Model file for the job. Use its own axes, mm. A direction names the side the tool comes from. Give positions to 0.01 mm unless a question says otherwise; leave off trailing zeros. Write each loop counter-clockwise with the first axis right and the second up, starting at its lowest first coordinate (ties: lowest second). Pieces come first, ordered by that corner, then holes. Notation, with made-up numbers: (27.25, -38.5) - (45.25, -38.5) arc R14 cw to (45.25, -30.5) - close; hole circle Ø11 at (-39.5, -27.5). An arc over 180 degrees is marked (long way). Use a Markdown table: item, result. Add a question column.
```python
from build123d import *

# Parameters (mm, degrees)
F1_DEPTH = 63.5
F0_W     = 25.4
F0_H     = 19.05
F2_DEPTH = 25.4
F3_DEPTH = 7.9375
F5_R     = 15.875


with BuildPart() as f1:
    # F0 (on Front) → F1 (new body, symmetric)
    with BuildSketch(Plane.XZ):
        Polygon((41.275, -9.525), (41.275, 9.525), (22.225, 9.525), (-41.275, 9.525), (-41.275, -9.525), align=None)
    extrude(amount=F1_DEPTH, both=True)

    # F0 (on Front) → F2 (join, symmetric)
    with BuildSketch(Plane.XZ):
        Polygon((41.275, -9.525), (41.275, 9.525), (22.225, 9.525), (-41.275, 9.525), (-41.275, -9.525), align=None)
        with BuildLine():
            Line((22.225, 9.525), (41.275, 9.525))
            Line((41.275, 9.525), (41.275, 27.0002))
            ThreePointArc((41.275, 27.0002), (45.9246798487, 38.2255201513), (57.15, 42.8752))
            Line((57.15, 42.8752), (60.325, 42.8752))
            Line((60.325, 42.8752), (60.325, 61.9252))
            Line((60.325, 61.9252), (57.15, 61.9252))
            ThreePointArc((57.15, 61.9252), (32.4542956671, 51.6959043329), (22.225, 27.0002))
            Line((22.225, 27.0002), (22.225, 9.525))
        make_face()
        with Locations((73.025, 52.4002)):
            Rectangle(F0_W, F0_H)
    extrude(amount=F2_DEPTH, both=True)

    # F0 (on Front) → F3 (join, symmetric)
    with BuildSketch(Plane.XZ):
        with BuildLine():
            Line((-41.275, 9.525), (22.225, 9.525))
            Line((22.225, 9.525), (22.225, 27.0002))
            ThreePointArc((22.225, 27.0002), (32.4542956671, 51.6959043329), (57.15, 61.9252))
            add(Edge.make_bspline(
                [(-41.275, 9.525), (-41.275, 34.925), (0, 61.9252), (57.15, 61.9252)],
                knots=[0, 0, 0, 0, 111.5045361635, 111.5045361635, 111.5045361635, 111.5045361635], degree=3))
        make_face()
    extrude(amount=F3_DEPTH, both=True)

    # F0 (on Front) → F4 (revolve)
    with BuildSketch(Plane.XZ):
        Polygon((85.725, 61.9252), (85.725, 42.8752), (85.725, 34.925), (111.125, 34.925), (111.125, 66.675), (85.725, 66.675), align=None)
    revolve(axis=Axis((85.725, 0, 50.8), (0, 0, -1)))

    # F5
    f5_edges = [f1.edges().sort_by_distance(p)[0] for p in [
        (41.275, -63.5, 0),
        (-41.275, -63.5, 0),
        (-41.275, 63.5, 0),
        (41.275, 63.5, 0),
    ]]
    fillet(f5_edges, radius=F5_R)


solid = f1.part
```
(1) Band-saw the part on B-B (y = -50). Write the cut outline in (x, z) (3 decimals).
(2) Two-plate mould, pull along X, no slides. Class faces 6 (the flat face through (60, 2, 42.875)), 7 (the cylindrical face through (36.748, 58.726, 0.133)), 8 (the cylindrical face through (32.73, -16.79, 51.97)): +X half, -X half, draft (parallel to the pull), parting line (faces both ways), or undercut.
(3) Flat gauge pins, fed straight in: pin 1 (1 mm diameter, centred on x = 63, y = 18, fed in from +Z); pin 2 (15.5 mm diameter, centred on x = 67, z = 45, fed in from +Y); pin 3 (3 mm diameter, centred on x = 75, z = 41, fed in from -Y). Where does each tip first touch, or does it go through?
(4) Probe probe 1 along X at (y, z) = (42.5, -6) (3 decimals); probe 2 along Y at (x, z) = (20.5, 44); probe 3 along Z at (x, y) = (-2.5, -54.5) (3 decimals). List the from-to ranges inside material, lowest first. Write a range as [from, to].
(5) Band-saw the part on A-A (y = 23). Write the cut outline in (x, z) (3 decimals).
(6) Which spindle directions (+Z, -Z, +X, -X, +Y, -Y) get a long thin tool onto all of the face, cutting with end or side? Do faces 1 (the flat face through (86, 0, 34.925)), 2 (the flat face through (46, -25.4, 42)), 3 (the flat face through (60, -2, 61.925)), 4 (the flat face through (46, 25.4, 42)), 5 (the flat face through (22.225, 17, 18)). Say none if no direction does.
Model answer:
| question | item | result |
|---|---|---|
| 1 | outline | (-41.096, -9.525) - (41.096, -9.525) - (41.096, 9.525) - (-41.096, 9.525) - close |
| 2 | face 6 | undercut |
| 2 | face 7 | +X half |
| 2 | face 8 | -X half |
| 3 | pin 1 | stops at z = 61.93 |
| 3 | pin 2 | stops at y = 25.4 |
| 3 | pin 3 | stops at y = -23.67 |
| 4 | probe 1 | x = [-41.275, 41.275] |
| 4 | probe 2 | y = [-7.94, 7.94] |
| 4 | probe 3 | z = [-9.525, 9.525] |
| 5 | outline | (-41.275, -9.525) - (41.275, -9.525) - (41.275, 27) arc R15.875 cw to (57.15, 42.875) - (74.947, 42.875) - (74.947, 34.925) - (96.503, 34.925) - (96.503, 66.675) - (74.947, 66.675) - (74.947, 61.925) - (57.15, 61.925) arc R34.925 ccw to (22.225, 27) - (22.225, 9.525) - (-41.275, 9.525) - close |
| 6 | face 1 | -Z, +X, +Y, -Y |
| 6 | face 2 | +Z, +X, -X, -Y |
| 6 | face 3 | +Z, -X |
| 6 | face 4 | +Z, +X, -X, +Y |
| 6 | face 5 | +Z, -X, +Y |
